Autodesk Inventor part; units mm, degrees
ref_plane "YZ Plane" through (0, 0, 0) normal (1, 0, 0) x (0, 1, 0)
ref_plane "XZ Plane" through (0, 0, 0) normal (0, 1, 0) x (-1, 0, 0)
ref_plane "XY Plane" through (0, 0, 0) normal (0, 0, 1) x (1, 0, 0)
sketch "Skizze1" plane through (0, 0, 0) normal (0, 0, 1) x (1, 0, 0)
  line L0 (-113.5762, 0) -> (48.979, 0)
  line L1 (0, -73.4285) -> (0, 160.1129)
  line L2 (-54.5088, -40.0654) -> (-14.5088, -40.0654)
  line L3 (-54.5088, -40.0654) -> (-54.5088, -10.0654)
  circle A0 centre (-54.5088, 109.9346) radius 10
  arc A1 (-14.5088, -40.0654) -> (-48.6674, 118.0511) centre (-89.0676, 26.5753) ccw
  arc A2 (-54.5088, -10.0654) -> (-60.3511, 101.8187) centre (-90.354, 44.1574) ccw
  point P0 (0, 0)
  point P1 (-58.162, 100.6258)
  dimension "d0" = 30
  dimension "d1" = 40
  dimension "d6" = 150
  dimension "d7" = 20
  dimension "d8" = 65
  dimension "d9" = 100
  dimension "d10" = 0
extrude "Extrusion1" add sketch "Skizze1" along normal blind 5 contours A2 A0 A1 L1 L0 | L0 L1 A1 L2 L3 A2 | L1 A1 L0 | L0 A1 L1 | A2 A0 picked at (-52.7779, 112.7657)
sketch "Skizze2" plane through (0, 0, 5) normal (0, 0, 1) x (1, 0, 0)
  arc A0 (-48.6674, 118.0511) -> (-60.3511, 101.8187) centre (-54.5088, 109.9346) ccw
  point P0 (0, 0)
  dimension "d13" = 0
  dimension "d14" = 0
hole "Bohrung1" at (-54.5088, 109.9346, 5) direction (0, 0, -1) diameter 3 end through all
sketch "Skizze3" plane through (0, 0, 5) normal (0, 0, 1) x (1, 0, 0)
  line L0 (-54.5088, -40.0654) -> (-14.5088, -40.0654)
  arc A0 (-54.5088, -10.0654) -> (-60.3511, 101.8187) centre (-90.354, 44.1574) ccw
  point P0 (0, 0)
  point P1 (-5.354, 49.9346)
  dimension "d22" = 90
  dimension "d23" = 85
hole "Bohrung2" at (-5.354, 49.9346, 5) direction (0, 0, -1) diameter 3 end through all
properties part number "Halterung hinten unten" material "Stahl"
Geometry check sheet. Reference: the model listing, model coordinates, mm. A direction names the side the tool comes from. Coordinates: 2 decimals unless noted, no trailing zeros. Order: outer loops, then holes, each group sorted by start corner. A loop starts at its lowest first (then second) coordinate and runs counter-clockwise, first axis right, second up.
Item 1: Section check B-B (z = 3.15). Enter the section's corners in (x, y).
Item 2: Tool access check on faces 1 (the cylindrical face through (-54.959, 108.504, 2.465)), 2 (the flat face through (-54.509, -25, 2)). Record the directions out of +Z, -Z, +X, -X, +Y, -Y that give a thin tool (end or side, any length) a straight path to the whole face; none if there is none.
Item 3: Section check A-A (x = -39). Enter the section's corners in (y, z).
Item 4: Scan lines: line 1 along X through (y, z) = (61, 1.3); line 2 along Y through (x, z) = (-44, 4.75); line 3 along Y through (x, z) = (-12, 3.85). Record each from-to range of solid material in increasing order.
Item 5: Section check D-D (x = -11). Enter the section's corners in (y, z).
Item 6: Mould release check, pull along Y, two halves, no side actions. Record for faces 3 (the cylindrical face through (-4.441, 51.125, 2.465)), 4 (the flat face through (-35, -40.065, 2)), 5 (the cylindrical face through (8.39, 48.98, 2.46)): released by +Y, released by -Y, zero draft, split by the parting line, or undercut.
Item 7: Section check C-C (y = 37). Enter the section's corners in (x, z).
Item 8: Depth check by flat-ended pin: pin 1 (1.5 mm diameter, centred on y = 55.5, z = 1, fed in from -X); pin 2 (2 mm diameter, centred on x = -18, z = 4, fed in from +Y); pin 3 (3 mm diameter, centred on y = 9, z = 4, fed in from +X). Enter the tip coordinate at first touch or a pass-through.
Check sheet entries:
1. outline: (-60.35, 101.82) arc R65 cw to (-54.51, -10.07) - (-54.51, -40.07) - (-14.51, -40.07) arc R100 ccw to (-48.67, 118.05) arc R10 ccw to start; hole circle Ø3 at (-54.51, 109.93); hole circle Ø3 at (-5.35, 49.93)
2. face 1: +Z, -Z
2. face 2: +Z, -Z, -X, -Y
3. outline: (-40.07, 0) - (4.31, 0) - (4.31, 5) - (-40.07, 5) - close; (84, 0) - (113.14, 0) - (113.14, 5) - (84, 5) - close
4. line 1: x = -27.57 to 4.82
4. line 2: y = -40.07 to -1.41, 89.72 to 115.84
4. line 3: y = -37.15 to 90.3
5. outline: (-35.92, 0) - (89.07, 0) - (89.07, 5) - (-35.92, 5) - close
6. face 3: undercut
6. face 4: released by -Y
6. face 5: split by the parting line
7. outline: (-25.75, 0) - (10.39, 0) - (10.39, 5) - (-25.75, 5) - close
8. pin 1: stops at x = -26.49
8. pin 2: stops at y = 97.92
8. pin 3: stops at x = 9.63
